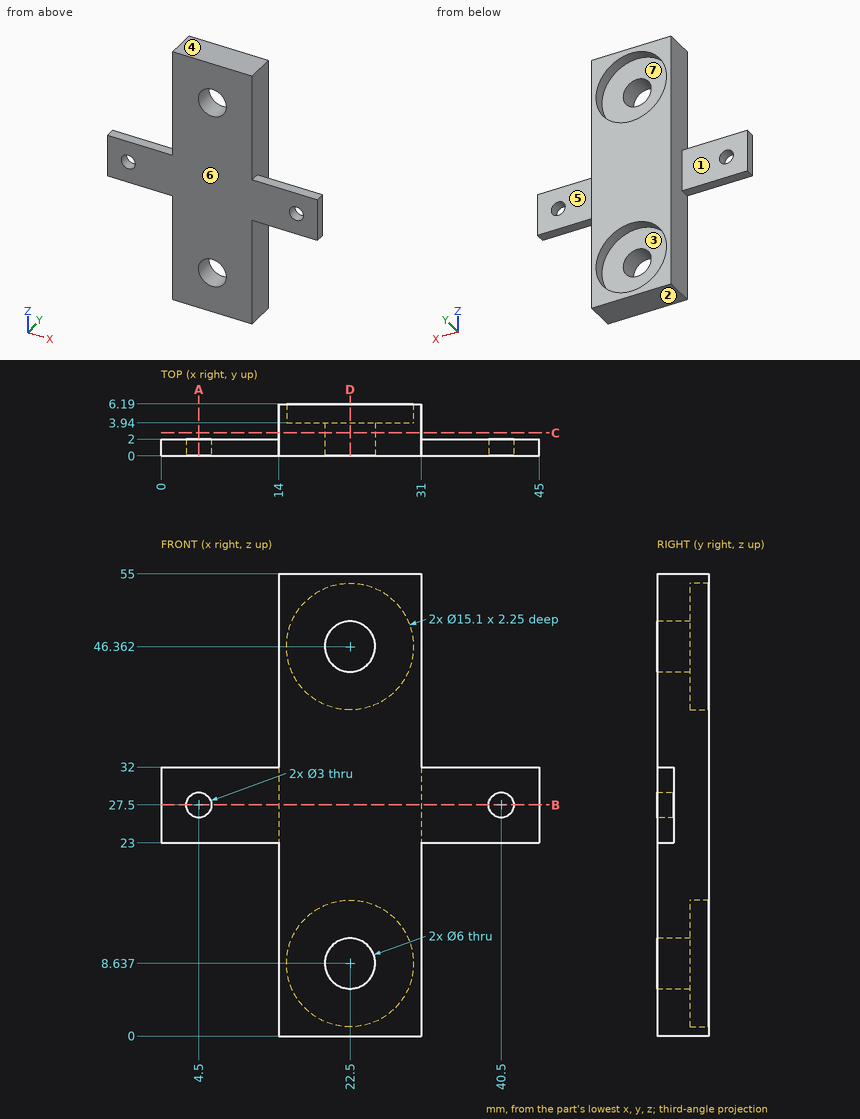
Could you check a few things on this drawing? It's one solid part, dimensions in mm from its lowest x, y, z. A direction names the side the tool comes from. Round coordinates to 2 decimals unless told otherwise and drop trailing zeros. Loops run counter-clockwise (first coordinate to the right, second up) from the corner with the lowest first, then second, coordinate; pieces in that order, holes last.
Q1. Please list where these lines run through material, in increasing order: L1, parallel to Z at x = 22.5, y = 5.7; L2, parallel to X at y = 1, z = 27.5; L3, parallel to Z at x = 28, y = 4.5 (1 decimal).
Q2. I want a section at B-B (z = 27.5). Write out the boundary of the cut face in (x, y), and give its area (3 significant figures).
Q3. For P1, Ø7, axis at x = 37.5, z = 27.5, coming from the +Y side; P2, Ø2, axis at x = 6, y = 1, coming from the +Z side; P3, Ø1.6, axis at x = 8, y = 1, coming from the -Z side, each with a flat end and sliding along its axis, tell me the tip position at first contact or that it passes through.
Q4. I want a section at A-A (x = 4.5). Write out the boundary of the cut face in (y, z), and give its area (3 significant figures).
Q5. I want a section at D-D (x = 22.5). Write out the boundary of the cut face in (y, z), and give its area (3 significant figures).
Q6. On a 3-axis mill with a long thin cutter (end or side, diameter ignored), from which of +Z, -Z, +X, -X, +Y, -Y can I reach the whole of each face in a straight line? I mean the marked faces 1, 2, 3, 4 and 5. Say none if no direction works.
Q7. Thinking about a two-plate mould opening in X: for the marked faces 6 and 7, which applies, pulls with the +X half, pulls with the -X half, needs draft (parallel to the pull), parting line crosses it, or undercut?
Q8. I want a section at C-C (y = 2.75). Write out the boundary of the cut face in (x, z).
Answer below:
1. L1: z = 0 to 1.09, 16.19 to 38.81, 53.91 to 55
1. L2: x = 0 to 3, 6 to 39, 42 to 45
1. L3: z = 0 to 3.5, 13.8 to 41.2, 51.5 to 55
2. outline: (0, 0) - (3, 0) - (3, 2) - (0, 2) - close; (6, 0) - (39, 0) - (39, 2) - (31, 2) - (31, 6.19) - (14, 6.19) - (14, 2) - (6, 2) - close; (42, 0) - (45, 0) - (45, 2) - (42, 2) - close
2. area: 149 mm2
3. P1: stops at y = 2
3. P2: stops at z = 32
3. P3: stops at z = 23
4. outline: (0, 23) - (2, 23) - (2, 26) - (0, 26) - close; (0, 29) - (2, 29) - (2, 32) - (0, 32) - close
4. area: 12.0 mm2
5. outline: (0, 0) - (6.19, 0) - (6.19, 1.09) - (3.94, 1.09) - (3.94, 5.64) - (0, 5.64) - close; (0, 11.64) - (3.94, 11.64) - (3.94, 16.19) - (6.19, 16.19) - (6.19, 38.81) - (3.94, 38.81) - (3.94, 43.36) - (0, 43.36) - close; (0, 49.36) - (3.94, 49.36) - (3.94, 53.91) - (6.19, 53.91) - (6.19, 55) - (0, 55) - close
5. area: 225 mm2
6. face 1: +Z, -Z, -X, +Y
6. face 2: -Z, +X, -X, +Y, -Y
6. face 3: +Y
6. face 4: +Z, +X, -X, +Y, -Y
6. face 5: +Z, -Z, +X, +Y
7. face 6: needs draft
7. face 7: undercut
8. outline: (14, 0) - (31, 0) - (31, 55) - (14, 55) - close; hole circle Ø6 at (22.5, 8.64); hole circle Ø6 at (22.5, 46.36)
